```python
from build123d import *

# Parameters (mm, degrees)
SKETCH_1_W          = 160.4
SKETCH_1_H          = 113
EXTRUDE_1_DEPTH     = 3
SKETCH_2_R          = 1.45
CUT_EXTRUDE_1_DEPTH = 3
SKETCH_3_R          = 23.297499696
CUT_EXTRUDE_2_DEPTH = 3
SKETCH_4_R          = 3
CUT_EXTRUDE_3_DEPTH = 3


with BuildPart() as part:
    # 草图1 → 凸台-拉伸1 (new body)
    with BuildSketch(Plane(origin=(0, 0, 0), x_dir=(1, 0, 0), z_dir=(0, 1, 0))):
        Rectangle(SKETCH_1_W, SKETCH_1_H)
    extrude(amount=EXTRUDE_1_DEPTH)

    # 草图2 → 切除-拉伸1 (cut)
    with BuildSketch(Plane(origin=(0, 3, 0), x_dir=(1, 0, 0), z_dir=(0, 1, 0))):
        with Locations(Location((0, -42.5, 0), (0, 0, 270))):
            Circle(SKETCH_2_R)
        with Locations(Location((-30.0520382, -30.0520382, 0), (0, 0, 270))):
            Circle(SKETCH_2_R)
        with Locations(Location((-42.5, 0, 0), (0, 0, 270))):
            Circle(SKETCH_2_R)
        with Locations(Location((-30.0520382, 30.0520382, 0), (0, 0, 270))):
            Circle(SKETCH_2_R)
        with Locations(Location((0, 42.5, 0), (0, 0, 270))):
            Circle(SKETCH_2_R)
        with Locations(Location((30.0520382, 30.0520382, 0), (0, 0, 270))):
            Circle(SKETCH_2_R)
        with Locations(Location((42.5, 0, 0), (0, 0, 270))):
            Circle(SKETCH_2_R)
        with Locations(Location((30.0520382, -30.0520382, 0), (0, 0, 270))):
            Circle(SKETCH_2_R)
    extrude(amount=-CUT_EXTRUDE_1_DEPTH, mode=Mode.SUBTRACT)

    # 草图3 → 切除-拉伸2 (cut)
    with BuildSketch(Plane.XZ):
        with Locations(Location((0, 0, 0), (0, 0, 270))):
            Circle(SKETCH_3_R)
    extrude(amount=-CUT_EXTRUDE_2_DEPTH, mode=Mode.SUBTRACT)

    # 草图4 → 切除-拉伸3 (cut)
    with BuildSketch(Plane(origin=(0, 3, 0), x_dir=(1, 0, 0), z_dir=(0, 1, 0))):
        with Locations(Location((70.198513237, -26.5, 0), (0, 0, 270))):
            Circle(SKETCH_4_R)
        with Locations(Location((-70.2, -26.5, 0), (0, 0, 270))):
            Circle(SKETCH_4_R)
        with Locations(Location((70.198513237, 26.5, 0), (0, 0, 270))):
            Circle(SKETCH_4_R)
        with Locations(Location((-70.2, 26.5, 0), (0, 0, 270))):
            Circle(SKETCH_4_R)
    extrude(amount=-CUT_EXTRUDE_3_DEPTH, mode=Mode.SUBTRACT)


solid = part.part
```
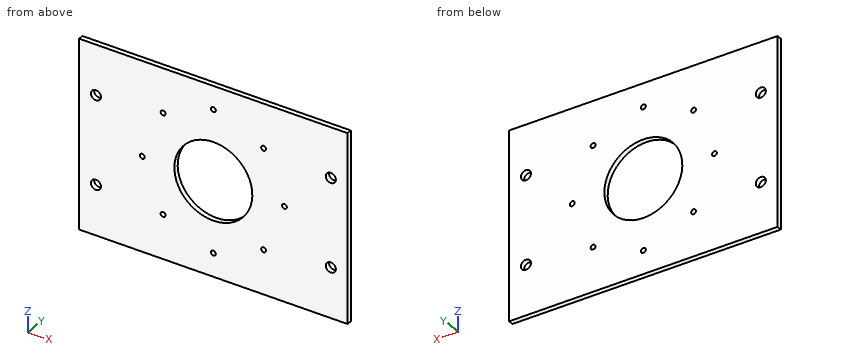
CAD build for the part. Positions are in the model's coordinates, mm. Round coordinates to 2 decimals unless told otherwise and drop trailing zeros. Loops run counter-clockwise (first coordinate to the right, second up) from the corner with the lowest first, then second, coordinate; pieces in that order, holes last. Notation, with made-up numbers: M -36,-1.5 L 4,-1.5 A11 ccw 4,8.5 Z; hole C 81,-22.75 d6. An arc over 180 degrees is marked long. Use a Markdown table: item, result. Add a question column.
(1) Drill centre lines: line 1 (X direction, y = 1.8, z = 0); line 2 (X direction, y = 0.7, z = -26.5); line 3 (Z direction, x = 1, y = 2.95). Where is each one in solid material? Low to high.
(2) Cut at C-C (y = 1.7). State how many separate pieces and enclosed holes the cut face has, and give its area (3 significant figures).
(3) Flat gauge pin, fed straight in: pin 1 (3.5 mm diameter, centred on x = 0, z = 42.5, fed in from +Y). Where does the tip first touch, or does it go through?
(4) Cut at B-B (x = -70.2). Give the cut face in (y, z), and give its area (3 significant figures).
(5) Cut at A-A (z = -26.5). Give the cut face in (x, y), and give its area (3 significant figures).
Geometry says:
| question | item | result |
|---|---|---|
| 1 | line 1 | x = -80.2 to -43.95, -41.05 to -23.3, 23.3 to 41.05, 43.95 to 80.2 |
| 1 | line 2 | x = -80.2 to -73.2, -67.2 to 67.2, 73.2 to 80.2 |
| 1 | line 3 | z = -56.5 to -43.55, -41.45 to -23.28, 23.28 to 41.45, 43.55 to 56.5 |
| 2 | separate pieces | 1 |
| 2 | enclosed holes | 13 |
| 2 | area | 16,300 mm² |
| 3 | pin 1 | stops at y = 3 |
| 4 | outline | M 0,-56.5 L 3,-56.5 L 3,-29.5 L 0,-29.5 Z; M 0,-23.5 L 3,-23.5 L 3,23.5 L 0,23.5 Z; M 0,29.5 L 3,29.5 L 3,56.5 L 0,56.5 Z |
| 4 | area | 303 mm² |
| 5 | outline | M -80.2,0 L -73.2,0 L -73.2,3 L -80.2,3 Z; M -67.2,0 L 67.2,0 L 67.2,3 L -67.2,3 Z; M 73.2,0 L 80.2,0 L 80.2,3 L 73.2,3 Z |
| 5 | area | 445 mm² |
